Source: CAD feature listing. Evaluate the final solid. Frame: model axes, mm. Face numbers are marked on the shaded views. A direction names the side the tool comes from. Give positions to 0.01 mm unless a question says otherwise; leave off trailing zeros. Loops run counter-clockwise (first coordinate to the right, second up) from the corner with the lowest first, then second, coordinate; pieces in that order, holes last. Notation, with made-up numbers: M -31.75,-8.5 L -4.75,-8.5 A22 ccw -4.75,7.5 Z; hole C 54.25,74 d5. An arc over 180 degrees is marked long. Put each result on its own line as item: value.
from build123d import *

# Parameters (mm, degrees)
F0_W      = 60
F0_H      = 30
F1_DEPTH  = 30
F2_R      = 14.99999
F3_SIZE   = 9
F4_R      = 7.5
F5_DEPTH  = 30
F6_W      = 9
F6_H      = 24
F6_W_2    = 18
F7_DEPTH  = 11.5
F8_START  = -18.5
F6_W_3    = 27
F8_DEPTH  = 11.501
F10_DEPTH = 7


# Not quite as in the source:
# - a fillet or chamfer is up to 0.001 mm smaller than in the source, because OpenCascade refuses the exact size


with BuildPart() as f1:
    # F0 (on Top) → F1 (new body)
    with BuildSketch(Plane.XY):
        with Locations((0, 0.9866876062)):
            Rectangle(F0_W, F0_H)
    extrude(amount=F1_DEPTH)

    # F2 (radius 15 in the source; OpenCascade refuses exactly that, so slightly less here)
    f2_edges = [f1.edges().sort_by_distance(p)[0] for p in [
        (-30, -14.013312, 15),
        (-30, 15.986688, 15),
    ]]
    fillet(f2_edges, radius=F2_R)

    # F3
    f3_edges = [f1.edges().sort_by_distance(p)[0] for p in [
        (30, -14.013312, 15),
        (30, 15.986688, 15),
    ]]
    chamfer(f3_edges, length=F3_SIZE)

    # F4 (on face) → F5 (cut, through all)
    with BuildSketch(Plane.XY.offset(30)):
        with Locations((-15, 0.9866876062)):
            Circle(F4_R)
    extrude(amount=-F5_DEPTH, mode=Mode.SUBTRACT)

    # F6 (on face) → F7 (cut)
    with BuildSketch(Plane.XZ.offset(14.0133123938)):
        with Locations((25.5, 18)):
            Rectangle(F6_W, F6_H)
        with Locations((12, 18)):
            Rectangle(F6_W_2, F6_H)
    extrude(amount=-F7_DEPTH, mode=Mode.SUBTRACT)

    # F6 (on face) → F8 (cut)
    with BuildSketch(Plane.XZ.offset(14.0133123938).offset(F8_START)):
        with Locations((16.5, 18)):
            Rectangle(F6_W_3, F6_H)
    extrude(amount=-F8_DEPTH, mode=Mode.SUBTRACT)

    # F9 (on face) → F10 (cut, through all)
    with BuildSketch(Plane.XZ.offset(2.5133123938)):
        Polygon((3, 30), (30, 6), (30, 30), align=None)
    extrude(amount=-F10_DEPTH, mode=Mode.SUBTRACT)


solid = f1.part
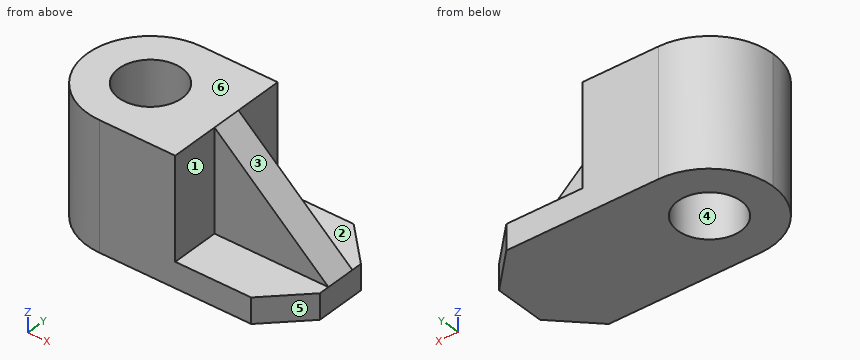
1. Section query C-C (x = 7.5). Output: boundary loops of the cut face in (y, z).
Found:
outline: M -14.01,0 L 15.99,0 L 15.99,6 L 4.49,6 L 4.49,26 L -2.51,26 L -2.51,6 L -14.01,6 Z
2. Draft query along X for the marked faces 4, 5 and 6. Return one class per face: pulls with the +X half, pulls with the -X half, needs draft (parallel to the pull), parting line crosses it, or undercut.
Found:
face 4: undercut
face 5: pulls with the +X half
face 6: needs draft
3. Section query A-A (y = 5.5). Output: boundary loops of the cut face in (x, z).
Found:
outline: M -29.3,0 L -20.99,0 L -20.99,30 L -29.3,30 Z; M -9.01,0 L 30,0 L 30,6 L 3,6 L 3,30 L -9.01,30 Z
4. Material intervals for line 1 (Y direction, x = -15, z = 6); line 2 (Y direction, x = 4, z = 10); line 3 (Z direction, x = 9.5, y = -3.5), sorted ascending. Write a range as from..to.
Found:
line 1: -14.01..-6.51, 8.49..15.99
line 2: -2.51..4.49
line 3: 0..6
5. Access query for the marked faces 1, 2 and 3. Directions: +Z, -Z, +X, -X, +Y, -Y. A direction counts if a zero-diameter tool reaches every point of the face in a straight line with its end or side. Return the directions, or none.
Found:
face 1: +Z, +X, -Y
face 2: +Z, +X, +Y
face 3: +Z, +X, +Y, -Y
6. Contact query for flat-ended pins moving along their axis: P1, Ø9, axis at y = -10.5, z = 23.5, coming from the +X side; P2, Ø12.5, axis at x = 16.5, y = -10.5, coming from the +Z side; P3, Ø12, axis at x = 13.5, z = 19.5, coming from the -Y side. Output: stop coordinate, or through.
Found:
P1: x = 3
P2: z = 6
P3: y = -2.51
